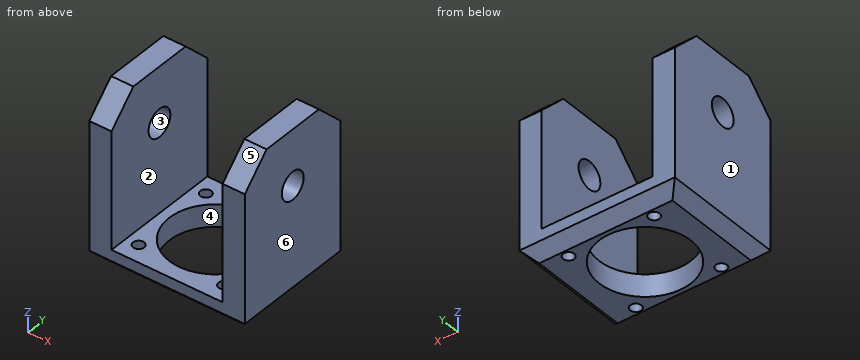
from build123d import *

# Parameters (mm, degrees)
SKETCH1_W           = 30
SKETCH1_H           = 22
BOSS_EXTRUDE1_DEPTH = 4
SKETCH2_W           = 4
SKETCH2_H           = 22
BOSS_EXTRUDE2_DEPTH = 20
SKETCH3_W           = 30
SKETCH3_H           = 22
BOSS_EXTRUDE3_DEPTH = 4
CHAMFER2_SIZE       = 5
SKETCH8_R           = 8.25
CUT_EXTRUDE1_DEPTH  = 4
SKETCH9_R           = 1
CUT_EXTRUDE2_DEPTH  = 4
CHAMFER3_SIZE       = 2
CUT_EXTRUDE3_REACH  = 48.562
SKETCH4_R           = 2.5


with BuildPart() as part:
    # Sketch1 → Boss-Extrude1 (new body)
    with BuildSketch(Plane(origin=(0, 0, 0), x_dir=(0, 0, -1), z_dir=(1, 0, 0))):
        with Locations((15, 11)):
            Rectangle(SKETCH1_W, SKETCH1_H)
    extrude(amount=BOSS_EXTRUDE1_DEPTH)

    # Sketch2 → Boss-Extrude2 (add)
    with BuildSketch(Plane.ZY):
        with Locations((-28, 11)):
            Rectangle(SKETCH2_W, SKETCH2_H)
    extrude(amount=BOSS_EXTRUDE2_DEPTH)

    # Sketch3 → Boss-Extrude3 (add)
    with BuildSketch(Plane.ZY.offset(20)):
        with Locations((-15, 11)):
            Rectangle(SKETCH3_W, SKETCH3_H)
    extrude(amount=BOSS_EXTRUDE3_DEPTH)

    # Chamfer2
    chamfer2_edges = [part.edges().sort_by_distance(p)[0] for p in [
        (-22, 22, 0),
        (-22, 0, 0),
        (2, 22, 0),
        (2, 0, 0),
    ]]
    chamfer(chamfer2_edges, length=CHAMFER2_SIZE)

    # Sketch8 → Cut-Extrude1 (cut)
    with BuildSketch(Plane.XY.offset(-26)):
        with Locations((-10, 11)):
            Circle(SKETCH8_R)
    extrude(amount=-CUT_EXTRUDE1_DEPTH, mode=Mode.SUBTRACT)

    # Sketch9 → Cut-Extrude2 (cut)
    with BuildSketch(Plane(origin=(0, 0, -30), x_dir=(-1, 0, 0), z_dir=(0, 0, -1))):
        with Locations((2.3, 18.7)):
            Circle(SKETCH9_R)
        with Locations((17.7, 18.7)):
            Circle(SKETCH9_R)
        with Locations((17.7, 3.3)):
            Circle(SKETCH9_R)
        with Locations((2.3, 3.3)):
            Circle(SKETCH9_R)
    extrude(amount=-CUT_EXTRUDE2_DEPTH, mode=Mode.SUBTRACT)

    # Chamfer3
    chamfer3_edges = [part.edges().sort_by_distance(p)[0] for p in [
        (4, 11, -30),
        (-24, 11, -30),
        (-10, 22, -30),
        (-10, 0, -30),
    ]]
    chamfer(chamfer3_edges, length=CHAMFER3_SIZE)

    # Cut-Extrude3: up to this face of the body (flat: up to its plane)
    cut_extrude3_end = Plane(part.part.faces().sort_by_distance((-24, 11, -14.521714608))[0])
    # Sketch4 → Cut-Extrude3 (cut, up to the picked face)
    with BuildSketch(Plane(origin=(4, 0, 0), x_dir=(0, 0, -1), z_dir=(1, 0, 0)), mode=Mode.PRIVATE) as cut_extrude3_sk1:
        with Locations(Location((10, 11, 0), (0, 0, 180))):
            Circle(SKETCH4_R)
    cut_extrude3_tool1 = split(extrude(cut_extrude3_sk1.sketch, amount=-CUT_EXTRUDE3_REACH, mode=Mode.PRIVATE), bisect_by=cut_extrude3_end, keep=Keep.BOTH, mode=Mode.PRIVATE)
    add(cut_extrude3_tool1.solids().sort_by(Axis((4, 11, -10), (-1, 0, 0)))[0], mode=Mode.SUBTRACT)


solid = part.part
Geometry: final body of the model. Coordinates: model frame, mm. Face numbers are marked on the shaded views. A direction names the side the tool comes from. Give positions to 0.01 mm unless a question says otherwise; leave off trailing zeros. Loops run counter-clockwise (first coordinate to the right, second up) from the corner with the lowest first, then second, coordinate; pieces in that order, holes last. Notation, with made-up numbers: (23.5, 15.25) - (57.5, 15.25) arc R15 ccw to (57.5, 30.25) - close; hole circle Ø9 at (61.25, 19.25). An arc over 180 degrees is marked (long way). Answer as CSV lines item,"result". Start each with the question number.
1. Draft query along Y for the marked faces 3, 4, 5 and 6. Return one class per face: released by +Y, released by -Y, zero draft, split by the parting line, or undercut.
2. Ray query, L1, parallel to Y at x = 2.9, z = -10; L2, parallel to X at y = 6.75, z = -25.5; L3, parallel to Y at x = -18.5, z = -27.5. Return the intervals inside material, ascending.
3. Pin query (flat end, axial travel): P1, Ø1.2, axis at x = -17.7, y = 18.7, coming from the +Z side; P2, Ø6, axis at x = -6, y = 16, coming from the +Z side; P3, Ø5, axis at x = -1, y = 17, coming from the +Z side. Return the tip coordinate at first contact, or that it passes through.
4. Section A-A, the plane z = -24. Return loops of the section in (x, y), plus the area to 3 significant figures.
5. Section B-B, the plane y = 3.3. Return loops of the section in (x, z).
6. Reachability of the marked faces 1 and 2 from +Z, -Z, +X, -X, +Y, -Y: full face, straight path, thin tool, end or side. Return the list, or none.
7. Section C-C, the plane x = -2.3. Return loops of the section in (y, z).
8. Section D-D, the plane z = -10. Return loops of the section in (x, y).
Answers:
1,face 3,"undercut"
1,face 4,"undercut"
1,face 5,"released by -Y"
1,face 6,"zero draft"
2,L1,"y = 0 to 8.5, 13.5 to 22"
2,L2,"x = -24 to -20, 0 to 4"
2,L3,"y = 0 to 2.7, 3.9 to 18.1, 19.3 to 22"
3,P1,"passes through"
3,P2,"stops at z = -26"
3,P3,"stops at z = 0"
4,outline,"(-24, 0) - (-20, 0) - (-20, 22) - (-24, 22) - close; (0, 0) - (4, 0) - (4, 22) - (0, 22) - close"
4,area,"176 mm2"
5,outline,"(-24, -28) - (-22, -30) - (-18.7, -30) - (-18.7, -26) - (-20, -26) - (-20, -1.7) - (-24, -1.7) - close; (-16.7, -30) - (-12.96, -30) - (-12.96, -26) - (-16.7, -26) - close; (-7.04, -30) - (-3.3, -30) - (-3.3, -26) - (-7.04, -26) - close; (-1.3, -30) - (2, -30) - (4, -28) - (4, -1.7) - (0, -1.7) - (0, -26) - (-1.3, -26) - close"
6,face 1,"+Z, -Z, -X, +Y, -Y"
6,face 2,"+Z, +Y, -Y"
7,outline,"(0, -28) - (2, -30) - (2.3, -30) - (2.3, -26) - (0, -26) - close; (4.3, -30) - (8.04, -30) - (8.04, -26) - (4.3, -26) - close; (13.96, -30) - (17.7, -30) - (17.7, -26) - (13.96, -26) - close; (19.7, -30) - (20, -30) - (22, -28) - (22, -26) - (19.7, -26) - close"
8,outline,"(-24, 0) - (-20, 0) - (-20, 8.5) - (-24, 8.5) - close; (-24, 13.5) - (-20, 13.5) - (-20, 22) - (-24, 22) - close; (0, 0) - (4, 0) - (4, 8.5) - (0, 8.5) - close; (0, 13.5) - (4, 13.5) - (4, 22) - (0, 22) - close"
